Autodesk Inventor part; units mm, degrees
ref_plane "YZ Plane" through (0, 0, 0) normal (1, 0, 0) x (0, 1, 0)
ref_plane "XZ Plane" through (0, 0, 0) normal (0, 1, 0) x (-1, 0, 0)
ref_plane "XY Plane" through (0, 0, 0) normal (0, 0, 1) x (1, 0, 0)
sketch "Sketch1" plane through (0, 0, 0) normal (0, 1, 0) x (-1, 0, 0)
  line L0 (0, 0) -> (-19.05, 0)
  line L1 (-19.05, 0) -> (-19.05, -273.05)
  line L2 (-19.05, -273.05) -> (0, -273.05)
  line L3 (0, -273.05) -> (0, 0)
  dimension "d0" = 19.05
  dimension "d1" = 273.05
extrude "Extrusion1" add sketch "Sketch1" along normal blind 3.175
sketch "Sketch4" plane through (19.05, 0, 0) normal (1, 0, 0) x (0, 0, -1)
  line L0 (273.05, 0) -> (273.05, 3.175)
  line L1 (0, 3.175) -> (273.05, 3.175)
  line L2 (273.05, 3.175) -> (273.05, 0)
  line L3 (273.05, 0) -> (0, 0)
  line L4 (0, 0) -> (0, 3.175)
extrude "Extrusion2" add sketch "Sketch4" along normal blind 6.35
sketch "Sketch5" plane through (0, 0, -273.05) normal (-1, 0, 0) x (0, 0, 1)
  line L0 (0, 0) -> (0, 3.175)
  line L1 (0, 3.175) -> (273.05, 3.175)
  line L2 (273.05, 3.175) -> (273.05, 0)
  line L3 (273.05, 0) -> (0, 0)
  line L4 (0, 0) -> (0, 3.175)
extrude "Extrusion3" add sketch "Sketch5" along normal blind 6.35
ref_plane "Work Plane1" through (9.525, 0, 0) normal (1, 0, 0) x (0, 0, -1)
ref_plane "Work Plane2" through (25.4, 0, -136.525) normal (0, 0, 1) x (1, 0, 0)
sketch "Sketch6" plane through (25.4, 0, 0) normal (1, 0, 0) x (0, 0, -1)
  line L0 (0, 0) -> (273.05, 0)
  line L1 (0, 3.175) -> (273.05, 3.175)
  line L2 (273.05, 3.175) -> (273.05, 0)
  line L3 (273.05, 0) -> (0, 0)
  line L4 (0, 0) -> (0, 3.175)
extrude "Extrusion4" add sketch "Sketch6" along normal blind 9.525
sketch "Sketch7" plane through (-6.35, 0, -273.05) normal (-1, 0, 0) x (0, 0, 1)
  line L0 (273.05, 3.175) -> (0, 3.175)
  line L1 (0, 3.175) -> (0, 0)
  line L2 (273.05, 3.175) -> (0, 3.175)
  line L3 (0, 3.175) -> (0, 0)
  line L4 (0, 0) -> (273.05, 0)
  line L5 (273.05, 0) -> (273.05, 3.175)
extrude "Extrusion5" add sketch "Sketch7" along normal blind 9.525
sketch "Sketch8" plane through (0, 3.175, 0) normal (0, 1, 0) x (1, 0, 0)
  line L0 (34.925, 273.05) -> (34.925, 0)
  line L1 (34.925, 0) -> (-15.875, 0)
  point P0 (0, 0)
  point P1 (30.1498, 124.6124)
  dimension "d30" = 4.7752
  dimension "d31" = 124.6124
hole "Hole3" at (30.1498, 3.175, -124.6124) direction (0, -1, 0) diameter 5.1816 end through all
mirror "Mirror4" about plane through (9.525, 0, 0) normal (1, 0, 0) of "Hole3"
mirror "Mirror5" about plane through (25.4, 0, -136.525) normal (0, 0, 1) of "Hole3", "Mirror4"
sketch "Sketch10" plane through (34.925, 0, 0) normal (1, 0, 0) x (0, 0, -1)
  line L0 (0, 3.175) -> (101.6, 3.175)
  line L1 (101.6, 3.175) -> (101.6, 0)
  line L2 (101.6, 0) -> (0, 0)
  line L3 (0, 0) -> (0, 3.175)
  dimension "d40" = 101.6
  dimension "d41" = 3.175
extrude "Extrusion6" cut sketch "Sketch10" against normal blind 15.875
chamfer "Chamfer1" distance 15.875 angle 45 1 edges at (19.05, 1.5875, -101.6)
mirror "Mirror6" about plane through (9.525, 0, 0) normal (1, 0, 0) of "Extrusion6", "Chamfer1"
mirror "Mirror7" about plane through (25.4, 0, -136.525) normal (0, 0, 1) of "Extrusion6", "Chamfer1", "Mirror6"
sketch "Sketch11" plane through (0, 3.175, 0) normal (0, 1, 0) x (1, 0, 0)
  line L0 (19.05, 0) -> (0, 0)
  line L1 (0, 85.725) -> (0, 0)
  point P0 (9.525, 16.2687)
  dimension "d47" = 16.2687
  dimension "d48" = 9.525
hole "Hole4" at (9.525, 3.175, -16.2687) direction (0, -1, 0) diameter 7.1374 end through all
mirror "Mirror8" about plane through (25.4, 0, -136.525) normal (0, 0, 1) of "Hole4"
properties part number "top beam"
Read the model definition and answer for the solid it produces. Units are mm, in the model's axes. Coordinates: 2 decimals unless noted, no trailing zeros. Write each loop counter-clockwise with the first axis right and the second up, starting at its lowest first coordinate (ties: lowest second). Pieces come first, ordered by that corner, then holes. Notation, with made-up numbers: (16.5, 80) -> (26.5, 80) arc R10 ccw to (26.5, 98) -> close; hole circle Ø7 at (71.25, 75.25). An arc over 180 degrees is marked (long way). Answer as a JSON object with one key per item and string values.
Q1. The part is cut by section A-A on y = 0.85. Give the number of separate pieces and of enclosed holes in the cut face, then the cut area to 3 significant figures.
The answers:
{"separate pieces": "1", "enclosed holes": "6", "area": "7,760 mm2"}
Q2. Consider line 1 (Z direction, x = 10, y = 0.7); line 2 (Z direction, x = 12, y = 1.6); line 3 (X direction, y = 0.95, z = -231.5). Determine where each line is inside the solid, lowest interval first. Write a range as [from, to].
The answers:
{"line 1": "z = [-273.05, -260.32], [-253.24, -19.81], [-12.73, 0]", "line 2": "z = [-273.05, -259.35], [-254.21, -18.84], [-13.7, 0]", "line 3": "x = [0, 19.05]"}
Q3. The part is cut by section C-C on x = -3. Give the vertices of the cut face in (y, z) (3 decimals).
The answers:
{"outline": "(0, -184.325) -> (3.175, -184.325) -> (3.175, -88.725) -> (0, -88.725) -> close"}
Q4. The part is cut by section B-B on z = -28. Give the vertices of the cut face in (x, y) (3 decimals), then the cut area to 3 significant figures.
The answers:
{"outline": "(0, 0) -> (19.05, 0) -> (19.05, 3.175) -> (0, 3.175) -> close", "area": "60.5 mm2"}
